```python
from build123d import *

# Parameters (mm, degrees)
SKETCH1_W               = 45
SKETCH1_H               = 159.1
BOSS_EXTRUDE1_DEPTH     = 115
SHELL1_T                = -2
CUT_EXTRUDE1_DEPTH      = 147.895209248
CUT_EXTRUDE1_DEPTH_BACK = 147.895209248
FILLET1_R               = 2
SKETCH3_W               = 36
SKETCH3_H               = 1
CUT_EXTRUDE2_DEPTH      = 4
LPATTERN1_COUNT         = 10
LPATTERN1_PITCH         = 3
SKETCH8_W               = 27.700077209
SKETCH8_H               = 1
CUT_EXTRUDE4_DEPTH      = 5
LPATTERN2_COUNT         = 10
LPATTERN2_PITCH         = 3
CUT_EXTRUDE3_DEPTH      = 147.895209411
SKETCH7_W               = 1
SKETCH7_H               = 6.5
BOSS_EXTRUDE3_DEPTH     = 90
CHAMFER2_SIZE           = 0.5
CUT_EXTRUDE6_DEPTH      = 9.105
SKETCH11_W              = 1
SKETCH11_H              = 6.5
BOSS_EXTRUDE6_DEPTH     = 89
SKETCH12_W              = 14.9796
SKETCH12_H              = 72.79
SKETCH12_W_2            = 14.049996967
SKETCH12_H_2            = 11.05
CUT_EXTRUDE7_DEPTH      = 2


with BuildPart() as part:
    # Sketch1 → Boss-Extrude1 (new body)
    with BuildSketch(Plane.XY):
        Rectangle(SKETCH1_W, SKETCH1_H)
    extrude(amount=BOSS_EXTRUDE1_DEPTH)

    # Shell1
    shell1_openings = [part.faces().sort_by_distance(p)[0] for p in [
        (0, 0, 115),
    ]]
    offset(amount=SHELL1_T, openings=shell1_openings, kind=Kind.INTERSECTION)

    # Sketch2 → Cut-Extrude1 (cut, two sides: drawn at the far end of the back side and taken through both)
    with BuildSketch(Plane(origin=(22.5, 0, 0), x_dir=(0, 0, -1), z_dir=(1, 0, 0)).offset(-CUT_EXTRUDE1_DEPTH_BACK)):
        with BuildLine():
            Line((-115, 482.170987722), (-115, 79.55))
            Line((-115, 79.55), (-115, 58.65))
            ThreePointArc((-115, 58.65), (-111.742842211, -10.755043044), (-102, -79.55))
            Line((-102, -79.55), (-26.918013628, -475.108282781))
            Line((-26.918013628, -475.108282781), (-828.772746701, -548.88921573))
            Line((-828.772746701, -548.88921573), (-916.854733073, 408.390054773))
            Line((-916.854733073, 408.390054773), (-115, 482.170987722))
        make_face()
    extrude(amount=CUT_EXTRUDE1_DEPTH + CUT_EXTRUDE1_DEPTH_BACK, mode=Mode.SUBTRACT)

    # Fillet1
    fillet1_edges = [part.edges().sort_by_distance(p)[0] for p in [
        (22.5, -79.55, 51),
        (-22.5, -79.55, 51),
        (-22.5, 79.55, 57.5),
        (22.5, 79.55, 57.5),
    ]]
    fillet(fillet1_edges, radius=FILLET1_R)

    # Sketch3 → Cut-Extrude2 (cut)
    with BuildSketch(Plane(origin=(0, 79.55, 0), x_dir=(1, 0, 0), z_dir=(0, 1, 0))):
        with Locations((0, -110)):
            Rectangle(SKETCH3_W, SKETCH3_H)
    cut_extrude2 = extrude(amount=-CUT_EXTRUDE2_DEPTH, mode=Mode.SUBTRACT)

    # LPattern1: Cut-Extrude2 ×10
    with Locations(*[(0, 0, -i * LPATTERN1_PITCH) for i in range(1, LPATTERN1_COUNT)]):
        add(cut_extrude2, mode=Mode.SUBTRACT)

    # Sketch8 → Cut-Extrude4 (cut)
    with BuildSketch(Plane.XZ.offset(79.55)):
        with Locations((0.524208986, 97.5)):
            Rectangle(SKETCH8_W, SKETCH8_H)
    cut_extrude4 = extrude(amount=-CUT_EXTRUDE4_DEPTH, mode=Mode.SUBTRACT)

    # LPattern2: Cut-Extrude4 ×10
    with Locations(*[(0, 0, -i * LPATTERN2_PITCH) for i in range(1, LPATTERN2_COUNT)]):
        add(cut_extrude4, mode=Mode.SUBTRACT)

    # Sketch5 → Cut-Extrude3 (cut, through all)
    with BuildSketch(Plane.ZY.offset(22.5)):
        with BuildLine():
            Line((65.347036406, 64.823533738), (66.838155653, 64.986516539))
            ThreePointArc((66.838155653, 64.986516539), (74.40797048, 34.807641847), (89.855449244, 7.799458383))
            Line((89.855449244, 7.799458383), (88.667189124, 6.88401429))
            ThreePointArc((88.667189124, 6.88401429), (73.01645406, 34.24756859), (65.347036406, 64.823533738))
        make_face()
        with BuildLine():
            Line((77.275990376, 66.127396149), (78.767109622, 66.29037895))
            ThreePointArc((78.767109622, 66.29037895), (84.83196797, 41.097147113), (97.049571899, 18.245197712))
            Line((97.049571899, 18.245197712), (95.827312392, 17.375668128))
            ThreePointArc((95.827312392, 17.375668128), (83.430037817, 40.563675608), (77.275990376, 66.127396149))
        make_face()
        with BuildLine():
            Line((89.204944346, 67.431258559), (90.696063592, 67.594241361))
            ThreePointArc((90.696063592, 67.594241361), (95.094328846, 47.99151385), (103.7314578, 29.852835107))
            Line((103.7314578, 29.852835107), (102.457595124, 29.060828868))
            ThreePointArc((102.457595124, 29.060828868), (93.67651402, 47.501818923), (89.204944346, 67.431258559))
        make_face()
    extrude(amount=-CUT_EXTRUDE3_DEPTH, mode=Mode.SUBTRACT)

    # Sketch7 → Boss-Extrude3 (add)
    with BuildSketch(Plane.XY.offset(95)):
        with Locations((-16, 74.3)):
            Rectangle(SKETCH7_W, SKETCH7_H)
        with Locations((-13.2, 74.3)):
            Rectangle(SKETCH7_W, SKETCH7_H)
    extrude(amount=-BOSS_EXTRUDE3_DEPTH)

    # Chamfer2
    chamfer2_edges = [part.edges().sort_by_distance(p)[0] for p in [
        (-13.7, 74.3, 95),
        (-15.5, 74.3, 95),
    ]]
    chamfer(chamfer2_edges, length=CHAMFER2_SIZE)

    # Sketch10 → Cut-Extrude6 (cut, symmetric)
    with BuildSketch(Plane(origin=(0, 0, 0), x_dir=(0, 0, -1), z_dir=(1, 0, 0))):
        with BuildLine():
            Line((-131.709183252, 78.35), (-112, 78.35))
            Line((-112, 78.35), (-112, 58.65))
            ThreePointArc((-112, 58.65), (-108.78648369, -10.149542881), (-99.173917094, -78.35))
            Line((-99.173917094, -78.35), (-102.923842912, -78.35))
            Line((-102.923842912, -78.35), (-131.709183252, 78.35))
        make_face()
    extrude(amount=CUT_EXTRUDE6_DEPTH, both=True, mode=Mode.SUBTRACT)

    # Sketch11 → Boss-Extrude6 (add)
    with BuildSketch(Plane.XY.offset(2)):
        with Locations((-16, -74.3)):
            Rectangle(SKETCH11_W, SKETCH11_H)
        with Locations((-13.2, -74.3)):
            Rectangle(SKETCH11_W, SKETCH11_H)
    extrude(amount=BOSS_EXTRUDE6_DEPTH)

    # Sketch12 → Cut-Extrude7 (cut)
    with BuildSketch(Plane(origin=(0, 0, 0), x_dir=(-1, 0, 0), z_dir=(0, 0, -1))):
        with Locations((8.5168, 0)):
            Rectangle(SKETCH12_W, SKETCH12_H)
        with Locations((10.674998484, -65.806322554)):
            Rectangle(SKETCH12_W_2, SKETCH12_H_2)
        with Locations((10.674998484, 65.795)):
            Rectangle(SKETCH12_W_2, SKETCH12_H_2)
    extrude(amount=-CUT_EXTRUDE7_DEPTH, mode=Mode.SUBTRACT)


solid = part.part
```
Read the model definition and answer for the solid it produces. Units are mm, in the model's axes. A direction names the side the tool comes from. Round coordinates to 2 decimals unless told otherwise and drop trailing zeros. Write each loop counter-clockwise with the first axis right and the second up, starting at its lowest first coordinate (ties: lowest second). Pieces come first, ordered by that corner, then holes. Notation, with made-up numbers: (78, 40) - (103, 40) arc R15 cw to (103, 65) - close; hole circle Ø9 at (15, 29). An arc over 180 degrees is marked (long way). Use CSV: the item, a comma, the result in double quotes.
Q1. Straight lines are drawn through the part: line 1 along Y through (x, z) = (13, 49); line 2 along X through (y, z) = (-56, 106); line 3 along Z through (x, y) = (7, -35.5). For each, find the intervals that lie inside material, in ascending order.
Values:
line 1,"y = -79.55 to -77.55, 77.55 to 79.55"
line 2,"x = -22.5 to -20.5, 20.5 to 22.5"
line 3,"z = 0 to 2"
Q2. Each of these flat-tipped pins is pushed along its axis until it touches: pin 1 Ø3 at (x, y) = (5, 44) entering from +Z; pin 2 Ø6 at (x, y) = (12.5, 46) entering from -Z; pin 3 Ø0.8 at (y, z) = (78.5, 110) entering from -X; pin 4 Ø1.1 at (y, z) = (-78.5, 70.5) entering from -X. Where does it stop, or does it pass through?
Values:
pin 1,"stops at z = 2"
pin 2,"stops at z = 0"
pin 3,"stops at x = -22.42"
pin 4,"stops at x = -22.46"
Q3. Find section A-A, the plane y = -66. Write down the section's boundary in (x, z), then the cut area to 3 significant figures.
Values:
outline,"(-22.5, 0) - (-17.7, 0) - (-17.7, 2) - (-20.5, 2) - (-20.5, 104.44) - (-22.5, 104.44) - close; (-3.65, 0) - (22.5, 0) - (22.5, 104.44) - (20.5, 104.44) - (20.5, 2) - (-3.65, 2) - close"
area,"472 mm²"
Q4. Find section C-C, the plane x = -6.5. Count the separate pieces of the cut face and the enclosed holes in it, then the cut area to 3 significant figures.
Values:
separate pieces,"24"
enclosed holes,"0"
area,"510 mm²"
Q5. Determine the mould class of faces 1 (the cylindrical face through (-21.772, -10.432, 111.773)), 2 (the cylindrical face through (-21.51, 48.26, 95)), 3 (the cylindrical face through (21.49, 47.23, 93.77)), 4 (the flat face through (0, 79, 115)) for opening direction Y: +Y half, -Y half, draft (parallel to the pull), parting line (faces both ways), or undercut.
Values:
face 1,"-Y half"
face 2,"undercut"
face 3,"undercut"
face 4,"draft"
Q6. Find section D-D, the plane y = -42.5. Write down the section's boundary in (x, z).
Values:
outline,"(-22.5, 0) - (22.5, 0) - (22.5, 108.06) - (20.5, 108.06) - (20.5, 2) - (-20.5, 2) - (-20.5, 108.06) - (-22.5, 108.06) - close"
Q7. A tool of negligible diameter and unlimited length cuts with its end or side. For faces 5 (the cylindrical face through (-21.51, 47.23, 93.77)), 6 (the flat face through (22.5, -1, 57)), 7 (the flat face through (-16.5, 74, 51)), from which of +Z, -Z, +X, -X, +Y, -Y can it reach the whole face along a straight path? Write none if from no direction.
Values:
face 5,"+X, -X"
face 6,"+Z, -Z, +X, +Y, -Y"
face 7,"+Z"
Q8. Find section B-B, the plane z = 7. Write down the section's boundary in (x, y).
Values:
outline,"(-22.5, -77.55) arc R2 ccw to (-20.5, -79.55) - (20.5, -79.55) arc R2 ccw to (22.5, -77.55) - (22.5, 77.55) arc R2 ccw to (20.5, 79.55) - (-20.5, 79.55) arc R2 ccw to (-22.5, 77.55) - close; hole (-20.5, -77.55) - (-16.5, -77.55) - (-16.5, -71.05) - (-15.5, -71.05) - (-15.5, -77.55) - (-13.7, -77.55) - (-13.7, -71.05) - (-12.7, -71.05) - (-12.7, -77.55) - (20.5, -77.55) - (20.5, 77.55) - (-12.7, 77.55) - (-12.7, 71.05) - (-13.7, 71.05) - (-13.7, 77.55) - (-15.5, 77.55) - (-15.5, 71.05) - (-16.5, 71.05) - (-16.5, 77.55) - (-20.5, 77.55) - close"
